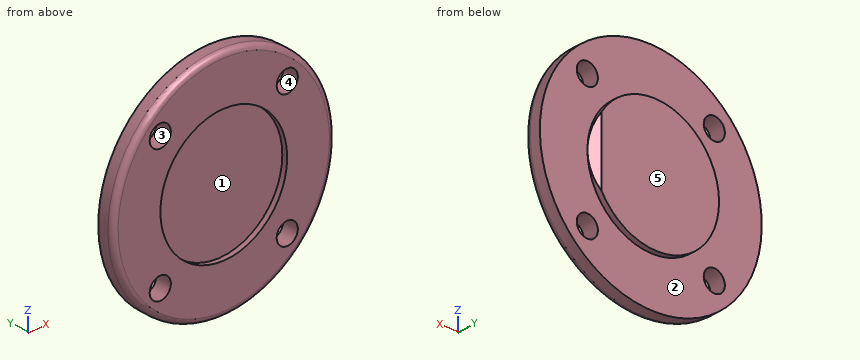
from build123d import *

# Parameters (mm, degrees)
SKETCH1_R           = 21
BOSS_EXTRUDE1_DEPTH = 3
SKETCH2_R           = 12
BOSS_EXTRUDE2_DEPTH = 1
CUT_EXTRUDE1_START  = -3
SKETCH2_2_R         = 12
CUT_EXTRUDE1_DEPTH  = 1
SKETCH3_R           = 2
CUT_EXTRUDE2_DEPTH  = 30.849623113
CIRPATTERN1_COUNT   = 4
FILLET1_R           = 1
CUT_EXTRUDE3_DEPTH  = 35.5


with BuildPart() as part:
    # Sketch1 → Boss-Extrude1 (new body)
    with BuildSketch(Plane(origin=(0, 0, 0), x_dir=(1, 0, 0), z_dir=(0, 1, 0))):
        with Locations(Location((0, 0, 0), (0, 0, 270))):
            Circle(SKETCH1_R)
    extrude(amount=BOSS_EXTRUDE1_DEPTH)

    # Sketch2 → Boss-Extrude2 (add)
    with BuildSketch(Plane(origin=(0, 3, 0), x_dir=(1, 0, 0), z_dir=(0, 1, 0))):
        with Locations(Location((0, 0, 0), (0, 0, 270))):
            Circle(SKETCH2_R)
    extrude(amount=BOSS_EXTRUDE2_DEPTH)

    # Sketch2_2 → Cut-Extrude1 (cut)
    with BuildSketch(Plane(origin=(0, 3, 0), x_dir=(1, 0, 0), z_dir=(0, 1, 0)).offset(CUT_EXTRUDE1_START)):
        with Locations(Location((0, 0, 0), (0, 0, 270))):
            Circle(SKETCH2_2_R)
    extrude(amount=CUT_EXTRUDE1_DEPTH, mode=Mode.SUBTRACT)

    # Sketch3 → Cut-Extrude2 (cut, through all)
    with BuildSketch(Plane(origin=(0, 3, 0), x_dir=(1, 0, 0), z_dir=(0, 1, 0))):
        with Locations(Location((12.02081528, 12.02081528, 0), (0, 0, 270))):
            Circle(SKETCH3_R)
    cut_extrude2 = extrude(amount=-CUT_EXTRUDE2_DEPTH, mode=Mode.SUBTRACT)

    # CirPattern1: Cut-Extrude2 ×4 about axis
    cirpattern1_axis = Axis((0, 0, 0), (0, 1, 0))
    for i in range(1, CIRPATTERN1_COUNT):
        add(cut_extrude2.rotate(cirpattern1_axis, i * 360 / CIRPATTERN1_COUNT), mode=Mode.SUBTRACT)

    # Fillet1
    fillet1_edges = [part.edges().sort_by_distance(p)[0] for p in [
        (0, 0, -21),
    ]]
    fillet(fillet1_edges, radius=FILLET1_R)

    # Sketch4 → Cut-Extrude3 (cut, symmetric)
    with BuildSketch(Plane.XY):
        Polygon((12, 3), (10.267949192, 4), (12, 4), align=None)
    extrude(amount=CUT_EXTRUDE3_DEPTH, both=True, mode=Mode.SUBTRACT)


solid = part.part
Verification items for the finished model (mm, model axes). Face numbers are marked on the shaded views. A direction names the side the tool comes from. Round coordinates to 2 decimals unless told otherwise and drop trailing zeros. Order: outer loops, then holes, each group sorted by start corner. A loop starts at its lowest first (then second) coordinate and runs counter-clockwise, first axis right, second up. Notation, with made-up numbers: (3.25, 28.25) -> (53.25, 28.25) arc R19 cw to (53.25, 56.25) -> close; hole circle Ø10 at (47, -10). An arc over 180 degrees is marked (long way). Put each result on its own line as item: value.
1) Mould release check, pull along Z, two halves, no side actions. Record for the marked faces 4 and 5: +Z half, -Z half, draft (parallel to the pull), parting line (faces both ways), or undercut.
Final values:
face 4: undercut
face 5: draft
2) Section check B-B (x = -13). Give the number of separate pieces and of enclosed holes in the cut face, then the cut area to 3 significant figures.
Final values:
separate pieces: 3
enclosed holes: 0
area: 77.5 mm^2
3) Material ranges on line 1 (Z direction, x = -11.5, y = 2.25); line 2 (Y direction, x = -10, z = -16); line 3 (X direction, y = 1.95, z = -13.5), recorded low to high.
Final values:
line 1: z = -17.57 to -13.95, -10.09 to 10.09, 13.95 to 17.57
line 2: y = 0 to 3
line 3: x = -16.09 to -13.37, -10.67 to 10.67, 13.37 to 16.09
4) Section check A-A (y = 1.85). Record the cut outline in (x, z).
Final values:
outline: circle Ø42 at (0, 0); hole circle Ø4 at (-12.02, -12.02); hole circle Ø4 at (-12.02, 12.02); hole circle Ø4 at (12.02, -12.02); hole circle Ø4 at (12.02, 12.02)
5) Depth check by flat-ended pin: pin 1 (1.5 mm diameter, centred on x = -3.5, y = 3.5, fed in from +Z); pin 2 (7 mm diameter, centred on x = -5.5, z = 0.5, fed in from -Y); pin 3 (6.5 mm diameter, centred on x = -12.02, z = -12.02, fed in from +Y). Enter the tip coordinate at first touch or a pass-through.
Final values:
pin 1: stops at z = 20.79
pin 2: stops at y = 1
pin 3: stops at y = 3
6) Set-up check for the marked faces 1, 2 and 3: record each of +Z, -Z, +X, -X, +Y, -Y from which the full face is reachable in a straight line by a thin tool's end or side.
Final values:
face 1: -Y
face 2: +Y
face 3: +Y, -Y
